The model under review builds one solid part; all positions refer to its coordinate system, in mm. Give positions to 0.01 mm unless a question says otherwise; leave off trailing zeros. Loops run counter-clockwise (first coordinate to the right, second up) from the corner with the lowest first, then second, coordinate; pieces in that order, holes last. Notation, with made-up numbers: M 45.25,45.5 L 77.25,45.5 A23 cw 77.25,83.5 Z; hole C -37.75,-28.75 d9. An arc over 180 degrees is marked long. Return JSON: item names as keys, results as strings.
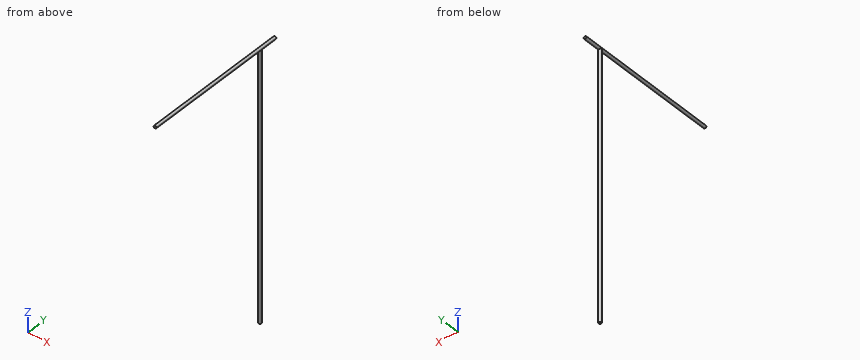
```python
from build123d import *

# Parameters (mm, degrees)
SKETCH_1_R           = 0.75
EXTRUDE_1_DEPTH      = 145
EXTRUDE_2_DEPTH      = 10
EXTRUDE_2_DEPTH_BACK = 70
SKETCH_2_R           = 0.75
MOVE_BODY_1_ANGLE    = 180


with BuildPart() as part:
    # 草图1 → 凸台-拉伸1 (new body)
    with BuildSketch(Plane.XY):
        Circle(SKETCH_1_R)
    extrude(amount=EXTRUDE_1_DEPTH)

    # 草图2 → 凸台-拉伸2 (add, two sides: drawn at the far end of the back side and taken through both)
    with BuildSketch(Plane(origin=(0, 0, 0), x_dir=(1, 0, 0), z_dir=(0, 1, 0)).offset(-EXTRUDE_2_DEPTH_BACK)):
        with Locations(Location((0, 0, 0), (0, 0, 270))):
            Circle(SKETCH_2_R)
    extrude(amount=EXTRUDE_2_DEPTH + EXTRUDE_2_DEPTH_BACK)


with BuildPart() as part_1:
    # Move Body 1: moved
    add(part.part.rotate(Axis((0, 0, 0), (0, 1, 0)), MOVE_BODY_1_ANGLE))


solid = part_1.part
```
1) Wall thickness on L1, parallel to Z at x = -0.2, y = 1; L2, parallel to Z at x = 0.4, y = -36.5: over which ranges is each line inside the solid? List them lowest first. Write a range as from..to.
From the geometry:
{"L1": "-0.72..0.72", "L2": "-0.63..0.63"}
2) Consider section A-A on x = 0. Write out the cut boundary in (y, z).
From the geometry:
{"outline": "M -70,-0.75 L -0.75,-0.75 L -0.75,-145 L 0.75,-145 L 0.75,-0.75 L 10,-0.75 L 10,0.75 L -70,0.75 Z"}
3) Consider section B-B on z = -16. Write out the cut boundary in (x, y), then the cut area to 3 significant figures.
From the geometry:
{"outline": "C 0,0 d1.5", "area": "1.77 mm²"}
